Design review of the part built by this model. Coordinates are the model's own, in mm. Face numbers are marked on the shaded views. A direction names the side the tool comes from. Give positions to 0.01 mm unless a question says otherwise; leave off trailing zeros. Loops run counter-clockwise (first coordinate to the right, second up) from the corner with the lowest first, then second, coordinate; pieces in that order, holes last. Notation, with made-up numbers: (-12.5, 74) - (-1.5, 74) arc R22 ccw to (-1.5, 109) - close; hole circle Ø1 at (36, 22). An arc over 180 degrees is marked (long way). Put each result on its own line as item: value. Start each with the question number.
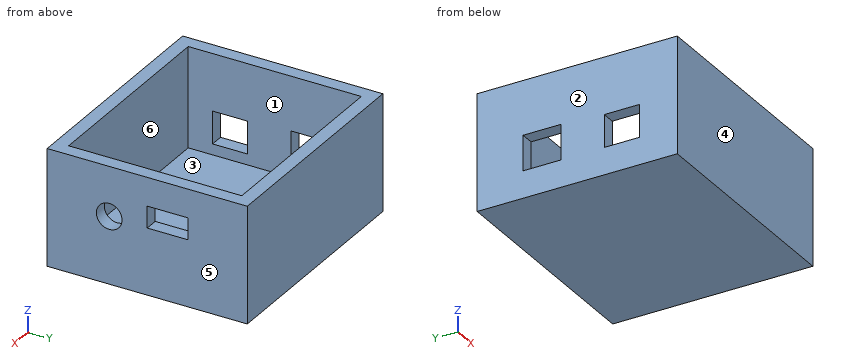
```python
from build123d import *

# Parameters (mm, degrees)
F0_W      = 85
F0_H      = 74
F1_DEPTH  = 43
F2_W      = 75
F2_H      = 64
F3_DEPTH  = 37
F4_W      = 15
F4_H      = 8
F5_DEPTH  = 6
F6_R      = 4.75
F7_DEPTH  = 6
F8_W      = 14
F8_H      = 13
F9_DEPTH  = 6
F10_W     = 13
F10_H     = 12
F11_DEPTH = 6


with BuildPart() as f1:
    # F0 (on Top) → F1 (new body)
    with BuildSketch(Plane.XY):
        Rectangle(F0_W, F0_H)
    extrude(amount=F1_DEPTH)

    # F2 (on face) → F3 (cut)
    with BuildSketch(Plane.XY.offset(43)):
        Rectangle(F2_W, F2_H)
    extrude(amount=-F3_DEPTH, mode=Mode.SUBTRACT)

    # F4 (on face) → F5 (cut)
    with BuildSketch(Plane.YZ.offset(42.5)):
        with Locations((7.5, 28.5)):
            Rectangle(F4_W, F4_H)
    extrude(amount=-F5_DEPTH, mode=Mode.SUBTRACT)

    # F6 (on face) → F7 (cut)
    with BuildSketch(Plane.YZ.offset(42.5)):
        with Locations((-14.05, 24.75)):
            Circle(F6_R)
    extrude(amount=-F7_DEPTH, mode=Mode.SUBTRACT)

    # F8 (on face) → F9 (cut)
    with BuildSketch(Plane(origin=(-42.5, 0, 0), x_dir=(0, -1, 0), z_dir=(-1, 0, 0))):
        with Locations((-13, 16.5)):
            Rectangle(F8_W, F8_H)
    extrude(amount=-F9_DEPTH, mode=Mode.SUBTRACT)

    # F10 (on face) → F11 (cut)
    with BuildSketch(Plane(origin=(-42.5, 0, 0), x_dir=(0, -1, 0), z_dir=(-1, 0, 0))):
        with Locations((16.5, 16)):
            Rectangle(F10_W, F10_H)
    extrude(amount=-F11_DEPTH, mode=Mode.SUBTRACT)


solid = f1.part
```
Item 1: For L1, parallel to X at y = -31, z = 27; L2, parallel to Z at x = 41.35, y = -14.05; L3, parallel to Y at x = -5, z = 30.5, list the stretches that pass through material, from the lowest coordinate up. Write a range as from..to.
Item 2: Mouldability with a two-part tool opening along X and no side actions: class the marked faces 3, 4, 5 and 6 as pulls with the +X half, pulls with the -X half, needs draft (parallel to the pull), parting line crosses it, or undercut.
Item 3: Consider section D-D (y = -31). State the section outline as (x, z) points, plus the area to 3 significant figures.
Item 4: Machinability: for the marked faces 1 and 2, which of the approach directions +Z, -Z, +X, -X, +Y, -Y give a long, thin tool a straight path to every point of the face, cutting with its end or side? Answer none if there is none.
Item 5: For P1, Ø19, axis at x = 4, y = -4, coming from the +Z side, flat-tipped, find the tip position at first contact; note if it passes through.
Item 6: Consider section C-C (x = 0). State the section outline as (y, z) points, plus the area to 3 significant figures.
Item 7: Consider section B-B (z = 11.5). State the section outline as (x, y) points, plus the area to 4 significant figures.
Item 8: Consider section A-A (y = -14.05). State the section outline as (x, z) points.
Geometry says:
1. L1: x = -42.5..-37.5, 37.5..42.5
1. L2: z = 0..20, 29.5..43
1. L3: y = -37..-32, 32..37
2. face 3: undercut
2. face 4: needs draft
2. face 5: pulls with the +X half
2. face 6: undercut
3. outline: (-42.5, 0) - (42.5, 0) - (42.5, 43) - (37.5, 43) - (37.5, 6) - (-37.5, 6) - (-37.5, 43) - (-42.5, 43) - close
3. area: 880 mm2
4. face 1: +Z
4. face 2: +Z, -Z, -X, +Y, -Y
5. P1: stops at z = 6
6. outline: (-37, 0) - (37, 0) - (37, 43) - (32, 43) - (32, 6) - (-32, 6) - (-32, 43) - (-37, 43) - close
6. area: 814 mm2
7. outline: (-42.5, -37) - (42.5, -37) - (42.5, 37) - (-42.5, 37) - (-42.5, 20) - (-37.5, 20) - (-37.5, 32) - (37.5, 32) - (37.5, -32) - (-37.5, -32) - (-37.5, -23) - (-42.5, -23) - close; (-42.5, -10) - (-37.5, -10) - (-37.5, 6) - (-42.5, 6) - close
7. area: 1,355 mm2
8. outline: (-42.5, 0) - (42.5, 0) - (42.5, 20) - (37.5, 20) - (37.5, 6) - (-37.5, 6) - (-37.5, 10) - (-42.5, 10) - close; (-42.5, 22) - (-37.5, 22) - (-37.5, 43) - (-42.5, 43) - close; (37.5, 29.5) - (42.5, 29.5) - (42.5, 43) - (37.5, 43) - close
